Design review of the part built by this model. Coordinates are the model's own, in mm. Face numbers are marked on the shaded views. A direction names the side the tool comes from. Give positions to 0.01 mm unless a question says otherwise; leave off trailing zeros. Loops run counter-clockwise (first coordinate to the right, second up) from the corner with the lowest first, then second, coordinate; pieces in that order, holes last. Notation, with made-up numbers: M 9,33 L 13,33 A20 cw 13,39 Z; hole C 42,10 d3. An arc over 180 degrees is marked long. Answer as CSV lines item,"result".
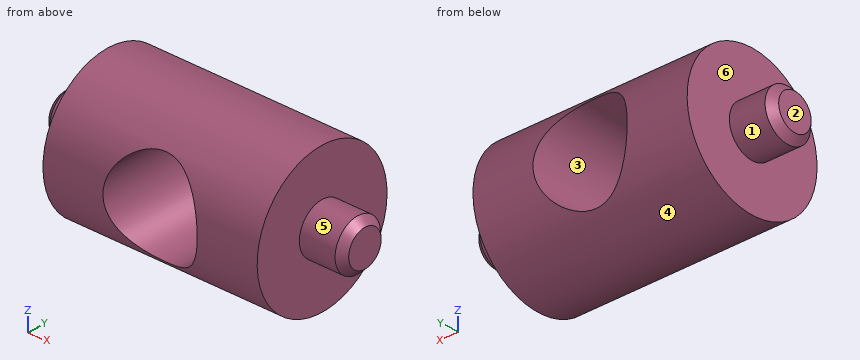
```python
from build123d import *

# Parameters (mm, degrees)
SMUSSO1_SIZE         = 0.5
FORO_PER_VITE_M6_2_D = 6.6


with BuildPart() as part:
    # Schizzo1 → Rivoluzione1 (revolve)
    with BuildSketch(Plane.XY, mode=Mode.PRIVATE) as rivoluzione1_sk:
        Polygon((-21, 0), (-21, 1.75), (-18, 1.75), (-18, 5), (-3, 5), (-3, 1.75), (0, 1.75), (0, 0), align=None)
    revolve(rivoluzione1_sk.sketch.rotate(Axis((-35.932586733, 0, 0), (1, 0, 0)), 90), axis=Axis((-35.932586733, 0, 0), (1, 0, 0)))

    # Smusso1
    smusso1_edges = [part.edges().sort_by_distance(p)[0] for p in [
        (0, 0, -1.75),
        (-21, 0, -1.75),
    ]]
    chamfer(smusso1_edges, length=SMUSSO1_SIZE)

    # Foro per Vite M6-2 (through all)
    with Locations(Plane(origin=(-10.5, 5, 0), x_dir=(0, 0, 1), z_dir=(0, 1, 0))):
        with Locations((0, 0)):
            Hole(FORO_PER_VITE_M6_2_D / 2)


solid = part.part
```
1. We need section C-C, the plane x = -9.75. Write out the cut boundary in (y, z).
Answer block:
outline,"M -3.83,-3.21 A5 ccw 3.83,-3.21 Z; M -3.83,3.21 L 3.83,3.21 A5 ccw Z"
2. To check wall thickness, follow L1, parallel to X at y = -1, z = 0; L2, parallel to Z at x = -8.5, y = -3.5; L3, parallel to X at y = 1.5, z = -1.75. State the ranges of each line that lie inside material, in increasing order. Write a range as [from, to].
Answer block:
L1,"[-21, -13.8], [-7.2, 0]"
L2,"[-3.57, -2.62], [2.62, 3.57]"
L3,"[-18, -13.3], [-7.7, -3]"
3. We need section D-D, the plane x = -17. Write out the cut boundary in (y, z), plus the area to 3 significant figures.
Answer block:
outline,"C 0,0 d10"
area,"78.5 mm²"
4. We need section B-B, the plane y = 0. Write out the cut boundary in (x, z), plus the area to 3 significant figures.
Answer block:
outline,"M -21,-1.25 L -20.5,-1.75 L -18,-1.75 L -18,-5 L -3,-5 L -3,-1.75 L -0.5,-1.75 L 0,-1.25 L 0,1.25 L -0.5,1.75 L -3,1.75 L -3,5 L -18,5 L -18,1.75 L -20.5,1.75 L -21,1.25 Z; hole C -10.5,0 d6.6"
area,"136 mm²"
5. We need section A-A, the plane z = 0. Write out the cut boundary in (x, y), plus the area to 4 significant figures.
Answer block:
outline,"M -21,-1.25 L -20.5,-1.75 L -18,-1.75 L -18,-5 L -13.8,-5 L -13.8,5 L -18,5 L -18,1.75 L -20.5,1.75 L -21,1.25 Z; M -7.2,-5 L -3,-5 L -3,-1.75 L -0.5,-1.75 L 0,-1.25 L 0,1.25 L -0.5,1.75 L -3,1.75 L -3,5 L -7.2,5 Z"
area,"104.5 mm²"
6. The part is to be moulded in two halves that separate along Z. For the marked faces 1, 2 and 3, say which applies: pulls with the +Z half, pulls with the -Z half, needs draft (parallel to the pull), parting line crosses it, or undercut.
Answer block:
face 1,"parting line crosses it"
face 2,"needs draft"
face 3,"undercut"
7. For the marked faces 4, 5 and 6, list the 3-axis set-ups (+Z, -Z, +X, -X, +Y, -Y) from which the entire face can be reached by the end or side of a thin tool; tool diameter is ignored.
Answer block:
face 4,"+X, -X"
face 5,"+X"
face 6,"-X"
